Read the model definition and answer for the solid it produces. Units are mm, in the model's axes. A direction names the side the tool comes from. Coordinates: 2 decimals unless noted, no trailing zeros. Write each loop counter-clockwise with the first axis right and the second up, starting at its lowest first coordinate (ties: lowest second). Pieces come first, ordered by that corner, then holes. Notation, with made-up numbers: (75.5, 84) - (132.5, 84) arc R25 cw to (132.5, 116) - close; hole circle Ø6 at (-28.5, 3). An arc over 180 degrees is marked (long way). Use a Markdown table: item, result.
from build123d import *

# Parameters (mm, degrees)
SKETCH1_R           = 101.6
BOSS_EXTRUDE1_DEPTH = 6.35
SCALE1_SCALE        = 0.4


with BuildPart() as part:
    # Sketch1 → Boss-Extrude1 (new body)
    with BuildSketch(Plane.XY):
        Circle(SKETCH1_R)
        with BuildLine():
            Line((-12.7, 14.199031657), (-12.7, 75.134213245))
            ThreePointArc((-12.7, 75.134213245), (-65.991135768, 38.1), (-71.418137364, -26.568583995))
            Line((-71.418137364, -26.568583995), (-18.646722124, 3.8990068))
            ThreePointArc((-18.646722124, 3.8990068), (-16.497783942, 9.525), (-12.7, 14.199031657))
        make_face(mode=Mode.SUBTRACT)
        with BuildLine():
            Line((12.7, 14.199031657), (12.7, 75.134213245))
            ThreePointArc((12.7, 75.134213245), (65.991135768, 38.1), (71.418137364, -26.568583995))
            Line((71.418137364, -26.568583995), (18.646722124, 3.8990068))
            ThreePointArc((18.646722124, 3.8990068), (16.497783942, 9.525), (12.7, 14.199031657))
        make_face(mode=Mode.SUBTRACT)
        with BuildLine():
            Line((5.946722124, -18.098038457), (58.718137364, -48.565629251))
            ThreePointArc((58.718137364, -48.565629251), (0, -76.2), (-58.718137364, -48.565629251))
            Line((-58.718137364, -48.565629251), (-5.946722124, -18.098038457))
            ThreePointArc((-5.946722124, -18.098038457), (0, -19.05), (5.946722124, -18.098038457))
        make_face(mode=Mode.SUBTRACT)
    extrude(amount=BOSS_EXTRUDE1_DEPTH)


with BuildPart() as part_1:
    # Scale1: scaled about (0, 0, 3.175)
    add(part.part.scale(SCALE1_SCALE).moved(Location((0, 0, 1.905))))


solid = part_1.part
(1) The mould has two halves that part along Y. Classify faces 1 (the cylindrical face through (-5.291, 40.294, 3.157)), 2 (the flat face through (-1, 1, 1.905)), 3 (the flat face through (18.16, -4.62, 3.16)): pulls with the +Y half, pulls with the -Y half, needs draft (parallel to the pull), parting line crosses it, or undercut.
Report:
| item | result |
|---|---|
| face 1 | parting line crosses it |
| face 2 | needs draft |
| face 3 | undercut |
(2) A cutting plane is placed at D-D, the plane y = -15.5. Write down the section's boundary in (x, z) (3 decimals), and give its area (3 significant figures).
Report:
| item | result |
|---|---|
| outline | (-37.568, 1.905) - (-16.687, 1.905) - (-16.687, 4.445) - (-37.568, 4.445) - close; (16.687, 1.905) - (37.568, 1.905) - (37.568, 4.445) - (16.687, 4.445) - close |
| area | 106 mm² |
(3) Straight lines are drawn through the part: L1, parallel to Y at x = 0.5, z = 2.8; L2, parallel to X at y = -3.5, z = 3.3; L3, parallel to X at y = 14, z = 3.25. For each, find the intervals that lie inside material, in ascending order.
Report:
| item | result |
|---|---|
| L1 | y = -40.64 to -30.48, -7.6 to 40.64 |
| L2 | x = -40.49 to -30.28, -16.22 to 16.22, 30.28 to 40.49 |
| L3 | x = -38.15 to -27.07, -5.08 to 5.08, 27.07 to 38.15 |
(4) A cutting plane is placed at C-C, the plane x = 0. Write down the section's boundary in (y, z) (3 decimals), and give its area (3 significant figures).
Report:
| item | result |
|---|---|
| outline | (-40.64, 1.905) - (-30.48, 1.905) - (-30.48, 4.445) - (-40.64, 4.445) - close; (-7.62, 1.905) - (40.64, 1.905) - (40.64, 4.445) - (-7.62, 4.445) - close |
| area | 148 mm² |
(5) Each of these flat-tipped pins is pushed along its axis until it touches: P1, Ø4, axis at x = 9, y = 15.5, coming from the +Z side; P2, Ø1.5, axis at y = 30, z = 3.5, coming from the +X side; P3, Ø1.3, axis at y = 16.5, z = 3.5, coming from the -X side; P4, Ø0.8, axis at y = 23, z = 3.5, coming from the +X side. Where does it stop, or does it pass through?
Report:
| item | result |
|---|---|
| P1 | passes through |
| P2 | stops at x = 28.21 |
| P3 | stops at x = -37.42 |
| P4 | stops at x = 33.78 |
(6) A cutting plane is placed at A-A, the plane z = 3.75. Write down the section's boundary in (x, y), and give its area (3 significant figures).
Report:
| item | result |
|---|---|
| outline | circle Ø81.28 at (0, 0); hole (-28.57, -10.63) - (-7.46, 1.56) arc R7.62 cw to (-5.08, 5.68) - (-5.08, 30.05) arc R30.48 ccw to start; hole (-23.49, -19.43) arc R30.48 ccw to (23.49, -19.43) - (2.38, -7.24) arc R7.62 cw to (-2.38, -7.24) - close; hole (5.08, 5.68) arc R7.62 cw to (7.46, 1.56) - (28.57, -10.63) arc R30.48 ccw to (5.08, 30.05) - close |
| area | 3,160 mm² |
(7) For faces 4 (the flat face through (-1, 1, 4.445)), 5 (the cylindrical face through (-0.03, -7.62, 3.16)), determine the directions among +Z, -Z, +X, -X, +Y, -Y from which every point of the face is accessible in a straight line to the end or side of a thin tool.
Report:
| item | result |
|---|---|
| face 4 | +Z, +X, -X, +Y, -Y |
| face 5 | +Z, -Z |
(8) A cutting plane is placed at B-B, the plane y = 0. Write down the section's boundary in (x, z) (3 decimals), and give its area (3 significant figures).
Report:
| item | result |
|---|---|
| outline | (-40.64, 1.905) - (-30.48, 1.905) - (-30.48, 4.445) - (-40.64, 4.445) - close; (-10.16, 1.905) - (10.16, 1.905) - (10.16, 4.445) - (-10.16, 4.445) - close; (30.48, 1.905) - (40.64, 1.905) - (40.64, 4.445) - (30.48, 4.445) - close |
| area | 103 mm² |
